Here's how the part is built. I have some questions about the finished solid (model axes, mm). A direction names the side the tool comes from. Round coordinates to 2 decimals unless told otherwise and drop trailing zeros. Write each loop counter-clockwise with the first axis right and the second up, starting at its lowest first coordinate (ties: lowest second). Pieces come first, ordered by that corner, then holes. Notation, with made-up numbers: (46, -10) - (65, -10) arc R20 ccw to (65, 17) - close; hole circle Ø5 at (41.25, -16.5). An arc over 180 degrees is marked (long way). One line per item, written item: value. Start each with the question number.
Item 1: If I drill on line 1 (Y direction, x = 222.5, z = 242); line 2 (X direction, y = 129.5, z = 830.5); line 3 (Z direction, x = -326.5, y = 162), over which ranges is the centre line in solid material (lowest first)?
Item 2: Imagine slicing it at A-A, the plane x = 72.5. Please give me the cut outline in (y, z), then the cut area to 3 significant figures.
Item 3: For faces 1 (the face through (348.74, 265.635, 1075.346)), 2 (the face through (-291.26, 110.787, 1149.104)), 3 (the face through (335, 430, -309)), 4 (the face through (-375.35, 127.05, 773.73)), 5 (the face through (375.35, 127.045, 42.24)), which set-ups out of +Z, -Z, +X, -X, +Y, -Y let a thin tool reach every point of the face, with its end or its side?
Item 4: Imagine slicing it at C-C, the plane y = 231.5. Please give me the cut outline in (x, z).
Item 5: Imagine slicing it at D-D, the plane y = 360.5. Please give me the cut outline in (x, z).
Item 6: Imagine slicing it at B-B, the plane z = 260. Please give me the cut outline in (x, y), then the cut area to 3 significant figures.
Item 7: For P1, Ø0.8, axis at x = 11, y = 343.5, coming from the -Z side; P2, Ø8, axis at x = 142.5, y = 383, coming from the -Z side; P3, Ø4, axis at x = 330, y = 416.5, coming from the +Z side; P4, Ø2, axis at x = -4, z = 837.5, coming from the -Y side, each with a flat end and sliding along its axis, tell me the tip position at first contact or that it passes through.
Item 8: Thinking about a two-plate mould opening in Y: for faces 6 (the face through (375, 47, 77.983)), 7 (the face through (330.14, 424.93, -323.07)), 8 (the face through (-375.35, 127.955, -125.26)), which applies, released by +Y, released by -Y, zero draft, split by the parting line, or undercut?
```python
from build123d import *

# Parameters (mm, degrees)
CROQUIS1_W              = 800
CROQUIS1_H              = 1600
SALIENTE_EXTRUIR1_DEPTH = 415
CORTAR_EXTRUIR1_DEPTH   = 200
CORTAR_EXTRUIR2_DEPTH   = 200
CORTAR_EXTRUIR6_DEPTH   = 499
CORTAR_EXTRUIR8_DEPTH   = 359
CORTAR_EXTRUIR10_DEPTH  = 353
CORTAR_EXTRUIR12_DEPTH  = 514
CORTAR_EXTRUIR13_DEPTH  = 514
CORTAR_EXTRUIR16_DEPTH  = 50
CORTAR_EXTRUIR17_DEPTH  = 50
CORTAR_EXTRUIR18_DEPTH  = 1
CROQUIS20_W             = 800
CROQUIS20_H             = 1
CORTAR_EXTRUIR19_DEPTH  = 1
SALIENTE_EXTRUIR2_DEPTH = 5
CROQUIS22_R             = 15
SALIENTE_EXTRUIR3_DEPTH = 10
CROQUIS23_R             = 20
SALIENTE_EXTRUIR4_DEPTH = 15
SALIENTE_EXTRUIR5_DEPTH = 5
CROQUIS26_R             = 25
SALIENTE_EXTRUIR6_DEPTH = 75


with BuildPart() as part:
    # Croquis1 → Saliente-Extruir1 (new body)
    with BuildSketch(Plane(origin=(0, 0, 0), x_dir=(1, 0, 0), z_dir=(0, 1, 0))):
        with Locations((0, -407.98258177)):
            Rectangle(CROQUIS1_W, CROQUIS1_H)
    extrude(amount=SALIENTE_EXTRUIR1_DEPTH)

    # Croquis3 → Cortar-Extruir1 (cut)
    with BuildSketch(Plane(origin=(604.100569287, 262.019524028, 906.150853931), x_dir=(-0.8421068082275548, 0.1498081502111445, 0.5180865194802076), z_dir=(-0.5393107856670403, -0.23391793113269235, -0.8089661785005605))):
        Polygon((456.118589156, 88.118028239), (242.368981337, -310.549885139), (242.368981337, 121.451272267), align=None)
    extrude(amount=-CORTAR_EXTRUIR1_DEPTH, mode=Mode.SUBTRACT)

    # Croquis5 → Cortar-Extruir2 (cut)
    with BuildSketch(Plane(origin=(-604.100569287, 262.019524028, 906.150853931), x_dir=(-0.8421068082275548, -0.1498081502111445, -0.5180865194802076), z_dir=(0.5393107856670404, -0.2339179311326923, -0.8089661785005605))):
        Polygon((-242.368981337, -310.549885139), (-242.368981337, 121.451272267), (-456.118589156, 88.118028239), align=None)
    extrude(amount=-CORTAR_EXTRUIR2_DEPTH, mode=Mode.SUBTRACT)

    # Croquis8 → Cortar-Extruir6 (cut)
    with BuildSketch(Plane(origin=(0, 250.204627362, 1153.721337281), x_dir=(-1, 0, 0), z_dir=(0, -0.21194078521367435, -0.9772825095963864))):
        Polygon((220, 168.626135247), (400, -256.020776905), (-400, -256.020776905), (-220, 168.626135247), (0, 168.626135247), align=None)
    extrude(amount=-CORTAR_EXTRUIR6_DEPTH, mode=Mode.SUBTRACT)

    # Croquis12 → Cortar-Extruir8 (cut)
    with BuildSketch(Plane.XY.offset(1117.98258177)):
        Polygon((220, 415), (400, 0), (400, 415), align=None)
    extrude(amount=CORTAR_EXTRUIR8_DEPTH, mode=Mode.SUBTRACT)

    # Croquis14 → Cortar-Extruir10 (cut)
    with BuildSketch(Plane.XY.offset(1117.98258177)):
        Polygon((-220, 415), (-400, 0), (-400, 415), align=None)
    extrude(amount=CORTAR_EXTRUIR10_DEPTH, mode=Mode.SUBTRACT)

    # Croquis15 → Cortar-Extruir12 (cut)
    with BuildSketch(Plane(origin=(516.98244579, 224.233349981, 1008.11576929), x_dir=(-0.8942171635698928, 0.0971910742249457, 0.4369548712029846), z_dir=(-0.44763340400043405, -0.19415424751826063, -0.8728851378008463))):
        Polygon((327.082120211, -262.279632659), (130.821069596, -242.738649788), (332.114454842, 162.361304614), align=None)
    extrude(amount=-CORTAR_EXTRUIR12_DEPTH, mode=Mode.SUBTRACT)


with BuildPart() as body_2:
    # of the pieces the cut leaves, the one that is kept (cortar_extruir12_keep)
    add(part.part.solids().sort_by_distance((-400, 0, 1207.98258177))[0])

    # Croquis16 → Cortar-Extruir13 (cut)
    with BuildSketch(Plane(origin=(-516.98244579, 224.233349981, 1008.11576929), x_dir=(-0.8942171635698928, -0.09719107422494568, -0.43695487120298454), z_dir=(0.44763340400043394, -0.19415424751826066, -0.8728851378008463))):
        Polygon((-327.082120211, -262.279632659), (-332.114454842, 162.361304614), (-130.821069596, -242.738649788), align=None)
    extrude(amount=-CORTAR_EXTRUIR13_DEPTH, mode=Mode.SUBTRACT)


with BuildPart() as body_2_2:
    # of the pieces the cut leaves, the one that is kept (cortar_extruir13_keep)
    add(body_2.part.solids().sort_by_distance((224.5, 0, 1207.98258177))[0])

    # Croquis17 → Cortar-Extruir16 (cut)
    with BuildSketch(Plane(origin=(400, 0, 0), x_dir=(0, 0, -1), z_dir=(1, 0, 0))):
        Polygon((162.01741823, 0), (-77.98258177, 0), (-77.98258177, 95), (-5.48258177, 160), (89.51741823, 160), (162.01741823, 95), align=None)
        Polygon((-977.98258177, 0), (-737.98258177, 0), (-737.98258177, 95), (-810.48258177, 160), (-905.48258177, 160), (-977.98258177, 95), align=None)
    extrude(amount=-CORTAR_EXTRUIR16_DEPTH, mode=Mode.SUBTRACT)

    # Croquis18 → Cortar-Extruir17 (cut)
    with BuildSketch(Plane.ZY.offset(400)):
        Polygon((-162.01741823, 0), (77.98258177, 0), (77.98258177, 95), (5.48258177, 160), (-89.51741823, 160), (-162.01741823, 95), align=None)
        Polygon((977.98258177, 0), (737.98258177, 0), (737.98258177, 95), (810.48258177, 160), (905.48258177, 160), (977.98258177, 95), align=None)
    extrude(amount=-CORTAR_EXTRUIR17_DEPTH, mode=Mode.SUBTRACT)

    # Croquis19 → Cortar-Extruir18 (cut)
    with BuildSketch(Plane(origin=(400, 0, 0), x_dir=(0, 0, -1), z_dir=(1, 0, 0))):
        Polygon((392.01741823, 343), (-948.718987098, 343), (-1091.223533976, 0), (-1092.306405756, 0), (-949.386393727, 344), (392.01741823, 344), align=None)
    cortar_extruir18 = extrude(amount=-CORTAR_EXTRUIR18_DEPTH, mode=Mode.SUBTRACT)

    # Croquis20 → Cortar-Extruir19 (cut)
    with BuildSketch(Plane(origin=(0, 0, -392.01741823), x_dir=(-1, 0, 0), z_dir=(0, 0, -1))):
        with Locations((0, 343.5)):
            Rectangle(CROQUIS20_W, CROQUIS20_H)
    extrude(amount=-CORTAR_EXTRUIR19_DEPTH, mode=Mode.SUBTRACT)

    # Simetr_a1: Cortar-Extruir18 across plane
    add(cortar_extruir18.mirror(Plane.ZY), mode=Mode.SUBTRACT)

    # Croquis21 → Saliente-Extruir2 (add)
    with BuildSketch(Plane(origin=(0, 415, 0), x_dir=(1, 0, 0), z_dir=(0, 1, 0))):
        with BuildLine():
            Line((295, 272.01741823), (345, 272.01741823))
            ThreePointArc((345, 272.01741823), (348.535533906, 273.481884325), (350, 277.01741823))
            Line((350, 277.01741823), (350, 347.01741823))
            ThreePointArc((350, 347.01741823), (348.535533906, 350.552952136), (345, 352.01741823))
            Line((345, 352.01741823), (295, 352.01741823))
            ThreePointArc((295, 352.01741823), (291.464466094, 350.552952136), (290, 347.01741823))
            Line((290, 347.01741823), (290, 277.01741823))
            ThreePointArc((290, 277.01741823), (291.464466094, 273.481884325), (295, 272.01741823))
        make_face()
        with BuildLine():
            Line((290, -882.98258177), (290, -952.98258177))
            ThreePointArc((290, -952.98258177), (291.464466094, -956.518115675), (295, -957.98258177))
            Line((295, -957.98258177), (345, -957.98258177))
            ThreePointArc((345, -957.98258177), (348.535533906, -956.518115675), (350, -952.98258177))
            Line((350, -952.98258177), (350, -882.98258177))
            ThreePointArc((350, -882.98258177), (348.535533906, -879.447047864), (345, -877.98258177))
            Line((345, -877.98258177), (295, -877.98258177))
            ThreePointArc((295, -877.98258177), (291.464466094, -879.447047864), (290, -882.98258177))
        make_face()
        with BuildLine():
            Line((-295, -877.98258177), (-345, -877.98258177))
            ThreePointArc((-345, -877.98258177), (-348.535533906, -879.447047864), (-350, -882.98258177))
            Line((-350, -882.98258177), (-350, -952.98258177))
            ThreePointArc((-350, -952.98258177), (-348.535533906, -956.518115675), (-345, -957.98258177))
            Line((-345, -957.98258177), (-295, -957.98258177))
            ThreePointArc((-295, -957.98258177), (-291.464466094, -956.518115675), (-290, -952.98258177))
            Line((-290, -952.98258177), (-290, -882.98258177))
            ThreePointArc((-290, -882.98258177), (-291.464466094, -879.447047864), (-295, -877.98258177))
        make_face()
    extrude(amount=SALIENTE_EXTRUIR2_DEPTH)

    # Croquis22 → Saliente-Extruir3 (add)
    with BuildSketch(Plane(origin=(0, 420, 0), x_dir=(1, 0, 0), z_dir=(0, 1, 0))):
        with Locations(Location((320, 312.01741823, 0), (0, 0, 270))):
            Circle(CROQUIS22_R)
        with Locations(Location((320, -917.98258177, 0), (0, 0, 270))):
            Circle(CROQUIS22_R)
        with Locations(Location((-320, -917.98258177, 0), (0, 0, 90))):
            Circle(CROQUIS22_R)
    extrude(amount=SALIENTE_EXTRUIR3_DEPTH)

    # Croquis23 → Saliente-Extruir4 (add)
    with BuildSketch(Plane(origin=(0, 430, 0), x_dir=(1, 0, 0), z_dir=(0, 1, 0))):
        with Locations(Location((320, 312.01741823, 0), (0, 0, 270))):
            Circle(CROQUIS23_R)
        with Locations(Location((320, -917.98258177, 0), (0, 0, 270))):
            Circle(CROQUIS23_R)
        with Locations(Location((-320, -917.98258177, 0), (0, 0, 270))):
            Circle(CROQUIS23_R)
    extrude(amount=SALIENTE_EXTRUIR4_DEPTH)

    # Croquis25 → Saliente-Extruir5 (add)
    with BuildSketch(Plane.XZ):
        with BuildLine():
            Line((-30, -476.764876907), (-30, -392.01741823))
            Line((-30, -392.01741823), (30, -392.01741823))
            Line((30, -392.01741823), (30, -476.764876907))
            ThreePointArc((30, -476.764876907), (0, -506.764876907), (-30, -476.764876907))
        make_face()
    extrude(amount=-SALIENTE_EXTRUIR5_DEPTH)

    # Croquis26 → Saliente-Extruir6 (add)
    with BuildSketch(Plane(origin=(0, 5, 0), x_dir=(1, 0, 0), z_dir=(0, 1, 0))):
        with Locations(Location((0, 476.764876907, 0), (0, 0, 90))):
            Circle(CROQUIS26_R)
    extrude(amount=SALIENTE_EXTRUIR6_DEPTH)

    # Croquis28 → Cortar-Revoluci_n7 (revolve, cut)
    with BuildSketch(Plane.ZY):
        with BuildLine():
            ThreePointArc((-451.764876907, 55), (-454.267783945, 44.096752398), (-461.275341569, 35.376690009))
            add(Edge.make_bspline(
                [(-461.275341569, 35.376690009), (-479.429840017, 14.56995995), (-453.764876907, 5)],
                knots=[0, 0, 0, 1, 1, 1], degree=2))
            Line((-453.764876907, 5), (-451.764876907, 5))
            Line((-451.764876907, 5), (-451.764876907, 55))
        make_face()
    revolve(axis=Axis((0, 90.386786237, -476.764876907), (0, -1, 0)), mode=Mode.SUBTRACT)

    # Croquis29 → Cortar-Revoluci_n26 (revolve, cut)
    with BuildSketch(Plane.ZY):
        with BuildLine():
            Line((-475.149447102, 80), (-475.149447102, 84.514502028))
            Line((-475.149447102, 84.514502028), (-446.334832781, 84.514502028))
            Line((-446.334832781, 84.514502028), (-446.334832781, 57.478552518))
            Line((-446.334832781, 57.478552518), (-451.764876907, 56.615429804))
            ThreePointArc((-451.764876907, 56.615429804), (-459.050340313, 72.714536594), (-475.149447102, 80))
        make_face()
    revolve(axis=Axis((0, 80, -476.764876907), (0, -1, 0)), mode=Mode.SUBTRACT)


solid = body_2_2.part
```
Values follow:
1. line 1: y = 0 to 415
1. line 2: x = -350 to 350
1. line 3: z = -392.02 to 1119.64
2. outline: (0, -392.02) - (343, -392.02) - (343, -391.02) - (344, -391.02) - (344, -392.02) - (415, -392.02) - (415, 1117.98) - (0, 1207.98) - close
2. area: 645,000 mm^2
3. face 1: +Z, +X, +Y
3. face 2: +Z, -X, +Y
3. face 3: none
3. face 4: -X, -Y
3. face 5: +X, -Y
4. outline: (-400, -392.02) - (400, -392.02) - (400, 995.04) - (399, 995.04) - (399, 996.13) - (400, 996.13) - (400, 1051.04) - (299.59, 1117.98) - (221.99, 1157.78) - (-221.99, 1157.78) - (-299.59, 1117.98) - (-400, 1051.04) - (-400, 996.13) - (-399, 996.13) - (-399, 995.04) - (-400, 995.04) - close
5. outline: (-400, -392.02) - (400, -392.02) - (400, 1013.74) - (243.64, 1117.98) - (220.59, 1129.8) - (-220.59, 1129.8) - (-243.64, 1117.98) - (-400, 1013.74) - close
6. outline: (-400, 0) - (400, 0) - (400, 343) - (399, 343) - (399, 344) - (400, 344) - (400, 415) - (-400, 415) - (-400, 344) - (-399, 344) - (-399, 343) - (-400, 343) - close
6. area: 332,000 mm^2
7. P1: stops at z = -391.02
7. P2: stops at z = -392.02
7. P3: stops at z = 1045.53
7. P4: stops at y = 0
8. face 6: zero draft
8. face 7: undercut
8. face 8: released by -Y
